Design review of the part built by this model. Coordinates are the model's own, in mm. A direction names the side the tool comes from. Coordinates: 2 decimals unless noted, no trailing zeros. Write each loop counter-clockwise with the first axis right and the second up, starting at its lowest first coordinate (ties: lowest second). Pieces come first, ordered by that corner, then holes. Notation, with made-up numbers: (43, 25) - (91, 25) arc R14 ccw to (91, 34) - close; hole circle Ø8 at (59.5, 85.25). An arc over 180 degrees is marked (long way). Answer as a JSON object with one key per item and string values.
```python
from build123d import *

# Parameters (mm, degrees)
SKETCH1_W                 = 65
SKETCH1_H                 = 10.18
BOSS_EXTRUDE1_DEPTH       = 3
F_5_0MM_DOWEL_HOLE1_D     = 5
F_5_0MM_DOWEL_HOLE1_DEPTH = 3
F_5_0MM_DOWEL_HOLE1_TIP   = 1.502151548
FILLET1_R                 = 5
SKETCH4_W                 = 3
SKETCH4_H                 = 4.91
CUT_EXTRUDE1_DEPTH        = 3


with BuildPart() as part:
    # Sketch1 → Boss-Extrude1 (new body)
    with BuildSketch(Plane(origin=(0, 0, 0), x_dir=(0, 0, -1), z_dir=(1, 0, 0))):
        with Locations((32.5, 5.09)):
            Rectangle(SKETCH1_W, SKETCH1_H)
    extrude(amount=BOSS_EXTRUDE1_DEPTH)

    # Ø5.0mm Dowel Hole1
    with Locations(Plane(origin=(3, 0, 0), x_dir=(0, 0, -1), z_dir=(1, 0, 0))):
        with Locations((10, 5.09)):
            Hole(F_5_0MM_DOWEL_HOLE1_D / 2, depth=F_5_0MM_DOWEL_HOLE1_DEPTH)
            with Locations((0, 0, -(F_5_0MM_DOWEL_HOLE1_DEPTH + F_5_0MM_DOWEL_HOLE1_TIP / 2))):  # 118° drill point
                Cone(0, F_5_0MM_DOWEL_HOLE1_D / 2, F_5_0MM_DOWEL_HOLE1_TIP, mode=Mode.SUBTRACT)

    # Fillet1
    fillet1_edges = [part.edges().sort_by_distance(p)[0] for p in [
        (1.5, 10.18, 0),
        (1.5, 0, 0),
    ]]
    fillet(fillet1_edges, radius=FILLET1_R)

    # Sketch4 → Cut-Extrude1 (cut)
    with BuildSketch(Plane(origin=(3, 0, 0), x_dir=(0, 0, -1), z_dir=(1, 0, 0))):
        with Locations((41.5, 5.09)):
            Rectangle(SKETCH4_W, SKETCH4_H)
    extrude(amount=-CUT_EXTRUDE1_DEPTH, mode=Mode.SUBTRACT)


solid = part.part
```
(1) Take a section at A-A, the plane z = -10. Write out the cut boundary in (x, y), and give its area (3 significant figures).
Solved:
{"outline": "(0, 0) - (3, 0) - (3, 2.59) - (0, 2.59) - close; (0, 7.59) - (3, 7.59) - (3, 10.18) - (0, 10.18) - close", "area": "15.5 mm^2"}
(2) The part is to be moulded in two halves that separate along Z. For faces 3 (the face through (1, 10.18, -35)), 4 (the face through (2, 2, -1)), 5 (the face through (2, 2.635, -41)), say which applies: pulls with the +Z half, pulls with the -Z half, needs draft (parallel to the pull), parting line crosses it, or undercut.
Solved:
{"face 3": "needs draft", "face 4": "pulls with the +Z half", "face 5": "undercut"}
(3) To check wall thickness, follow line 1 (Z direction, x = 0.8, y = 5.09); line 2 (Y direction, x = 1.6, z = -10); line 3 (Z direction, x = 2.85, y = 4). State the ranges of each line that lie inside material, in increasing order. Write a range as from..to.
Solved:
{"line 1": "z = -65..-43, -40..-12.5, -7.5..0", "line 2": "y = 0..2.59, 7.59..10.18", "line 3": "z = -65..-43, -40..-12.25, -7.75..-0.1"}
(4) Tool access review of faces 1 (the face through (3, 5, -32)), 2 (the face through (2, 5, -43)): name each direction out of +Z, -Z, +X, -X, +Y, -Y from which nothing blocks a thin tool from reaching the whole face with its end or side.
Solved:
{"face 1": "+Z, -Z, +X, +Y, -Y", "face 2": "+X, -X"}
(5) For pin 1 (4.5 mm diameter, centred on y = 5.09, z = -10, fed in from +X), flat-tipped, find the tip position at first contact; note if it passes through.
Solved:
{"pin 1": "passes through"}
(6) Take a section at B-B, the plane x = 1.85. Write out the cut boundary in (y, z) (3 decimals), and give its area (3 significant figures).
Solved:
{"outline": "(0, -65) - (10.18, -65) - (10.18, -5) arc R5 ccw to (5.18, 0) - (5, 0) arc R5 ccw to (0, -5) - close; hole circle Ø5 at (5.09, -10); hole (2.635, -43) - (7.545, -43) - (7.545, -40) - (2.635, -40) - close", "area": "617 mm^2"}
(7) Take a section at D-D, the plane y = 1.25. Write out the cut boundary in (x, z).
Solved:
{"outline": "(0, -65) - (3, -65) - (3, -1.69) - (0, -1.69) - close"}
(8) Take a section at C-C, the plane y = 3.75. Write out the cut boundary in (x, z).
Solved:
{"outline": "(0, -65) - (3, -65) - (3, -43) - (0, -43) - close; (0, -40) - (3, -40) - (3, -12.11) - (0, -12.11) - close; (0, -7.89) - (3, -7.89) - (3, -0.16) - (0, -0.16) - close"}
